Study the drawing (mm; zero at the part's minimum x, y, z) and answer. A direction names the side the tool comes from. Give positions to 0.01 mm unless a question says otherwise; leave off trailing zeros. Order: outer loops, then holes, each group sorted by start corner. A loop starts at its lowest first (then second) coordinate and runs counter-clockwise, first axis right, second up. Notation, with made-up numbers: (18.5, 62) - (76.5, 62) arc R10 cw to (76.5, 73) - close; hole circle Ø6 at (34.25, 59.5). An arc over 180 degrees is marked (long way). Return JSON: item names as keys, results as strings.
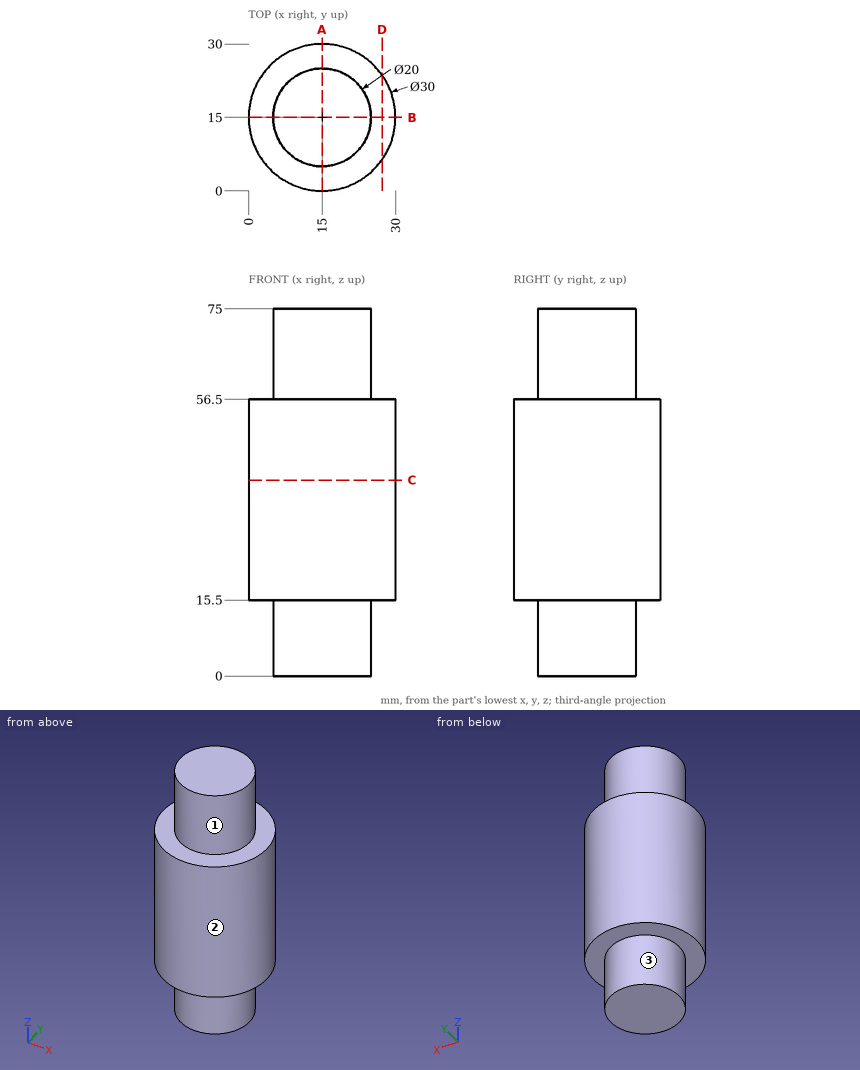
Q1. A cutting plane is placed at C-C (z = 40). Write down the section's boundary in (x, y).
Values:
{"outline": "circle Ø30 at (15, 15)"}
Q2. For the marked faces 1, 2 and 3, determine the directions among +Z, -Z, +X, -X, +Y, -Y from which every point of the face is accessible in a straight line to the end or side of a thin tool.
Values:
{"face 1": "+Z", "face 2": "+Z, -Z", "face 3": "-Z"}
Q3. A cutting plane is placed at A-A (x = 15). Write down the section's boundary in (y, z), and give its area (3 significant figures).
Values:
{"outline": "(0, 15.5) - (5, 15.5) - (5, 0) - (25, 0) - (25, 15.5) - (30, 15.5) - (30, 56.5) - (25, 56.5) - (25, 75) - (5, 75) - (5, 56.5) - (0, 56.5) - close", "area": "1,910 mm²"}
Q4. Consider L1, parallel to Z at x = 28, y = 18; L2, parallel to Y at x = 22.75, z = 25.5; L3, parallel to X at y = 7.5, z = 15. Determine where each line is inside the solid, lowest interval first.
Values:
{"L1": "z = 15.5 to 56.5", "L2": "y = 2.16 to 27.84", "L3": "x = 8.39 to 21.61"}
Q5. Given pin 1 (5 mm diameter, centred on y = 3, z = 14.5, fed in from -X); pin 2 (8 mm diameter, centred on x = 14, z = 48.5, fed in from -Y); pin 3 (4 mm diameter, centred on y = 7.5, z = 9.5, fed in from +X); pin 4 (3 mm diameter, centred on x = 12, z = 62.5, fed in from +Y), each flat-ended and moving along its own axis, determine where each tip first touches the part or whether it passes through.
Values:
{"pin 1": "stops at x = 3.57", "pin 2": "stops at y = 0", "pin 3": "stops at x = 23.35", "pin 4": "stops at y = 24.89"}
Q6. A cutting plane is placed at D-D (x = 27.25). Write down the section's boundary in (y, z), and give its area (3 significant figures).
Values:
{"outline": "(6.34, 15.5) - (23.66, 15.5) - (23.66, 56.5) - (6.34, 56.5) - close", "area": "710 mm²"}
